Answer from the drawing. Dimensions are ordinates in mm from the lowest x, y and z of the part. Coordinates: 2 decimals unless noted, no trailing zeros. Write each loop counter-clockwise with the first axis right and the second up, starting at its lowest first coordinate (ties: lowest second). Pieces come first, ordered by that corner, then holes.
(1) The part is cut by section B-B on x = 103. Determine the outline of the cut face in (y, z) (1 decimal), plus the area to 3 significant figures.
(2) Given P1, Ø3, axis at x = 65.5, y = 6, coming from the +Z side (1 decimal); P2, Ø1, axis at x = 28.5, y = 6, coming from the +Z side; P3, Ø6, axis at x = 65, y = 6.5, coming from the +Z side (1 decimal), each flat-ended and moving along its own axis, determine where each tip first touches the part or whether it passes through.
(3) The part is cut by section A-A on y = 2.5. Determine the outline of the cut face in (x, z).
(4) Straight lines are drawn through the part: line 1 (X direction, y = 3, z = 265) (1 decimal); line 2 (X direction, y = 4, z = 283.5); line 3 (Z direction, x = 60, y = 4.5) (1 decimal). For each, find the intervals that lie inside material, in ascending order.
(5) The part is cut by section D-D on z = 262. Determine the outline of the cut face in (x, y).
(6) The part is cut by section C-C on z = 454. Determine the outline of the cut face in (x, y) (1 decimal), plus the area to 3 significant figures.
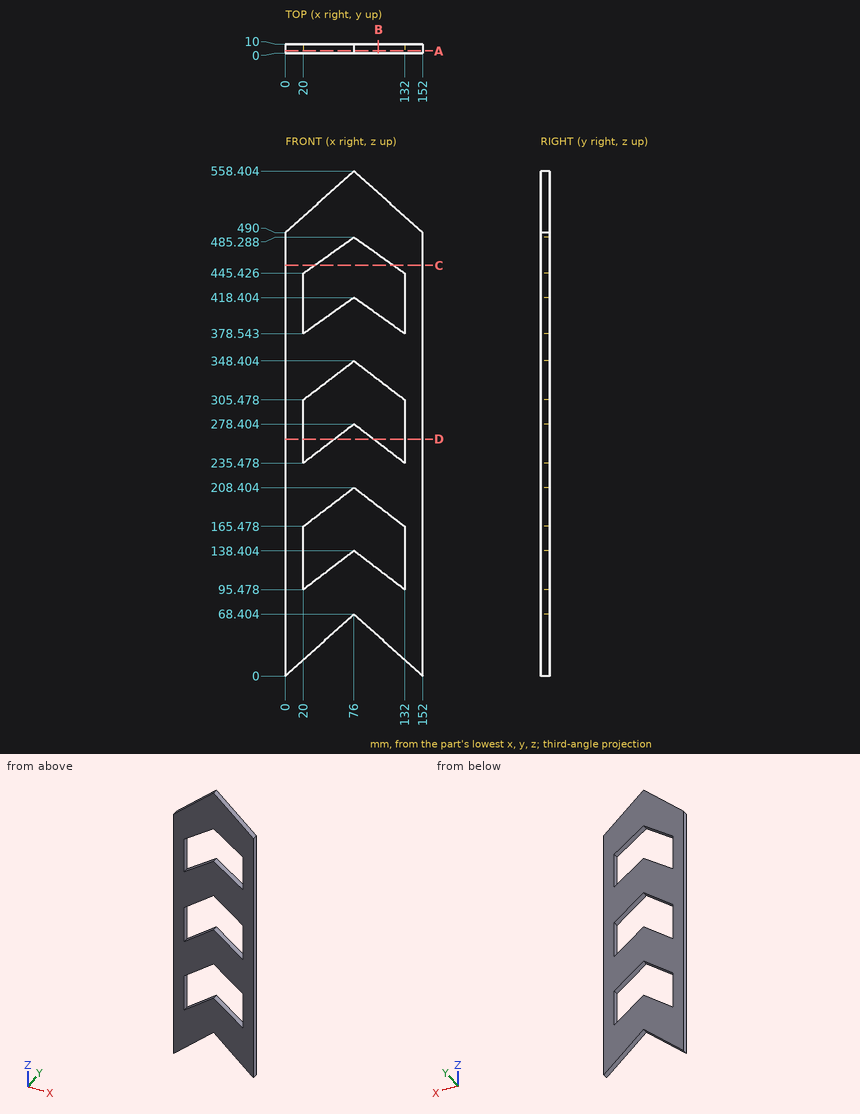
Model answer:
1. outline: (0, 44.1) - (10, 44.1) - (10, 117.7) - (0, 117.7) - close; (0, 187.7) - (10, 187.7) - (10, 257.7) - (0, 257.7) - close; (0, 327.7) - (10, 327.7) - (10, 399.2) - (0, 399.2) - close; (0, 466.1) - (10, 466.1) - (10, 534.1) - (0, 534.1) - close
1. area: 2,830 mm2
2. P1: stops at z = 550.3
2. P2: stops at z = 516.1
2. P3: stops at z = 551.2
3. outline: (0, 0) - (76, 68.4) - (152, 0) - (152, 490) - (76, 558.4) - (0, 490) - close; hole (20, 95.48) - (76, 138.4) - (132, 95.48) - (132, 165.48) - (76, 208.4) - (20, 165.48) - close; hole (20, 235.48) - (76, 278.4) - (132, 235.48) - (132, 305.48) - (76, 348.4) - (20, 305.48) - close; hole (20, 378.54) - (76, 418.4) - (132, 378.54) - (132, 445.43) - (76, 485.29) - (20, 445.43) - close
4. line 1: x = 0 to 20, 58.5 to 93.5, 132 to 152
4. line 2: x = 0 to 20, 132 to 152
4. line 3: z = 54 to 126.1, 196.1 to 266.1, 336.1 to 407, 473.9 to 544
5. outline: (0, 0) - (20, 0) - (20, 10) - (0, 10) - close; (54.6, 0) - (97.4, 0) - (97.4, 10) - (54.6, 10) - close; (132, 0) - (152, 0) - (152, 10) - (132, 10) - close
6. outline: (0, 0) - (32, 0) - (32, 10) - (0, 10) - close; (120, 0) - (152, 0) - (152, 10) - (120, 10) - close
6. area: 641 mm2
